Read the model definition and answer for the solid it produces. Units are mm, in the model's axes. Face numbers are marked on the shaded views. A direction names the side the tool comes from. Round coordinates to 2 decimals unless told otherwise and drop trailing zeros. Loops run counter-clockwise (first coordinate to the right, second up) from the corner with the lowest first, then second, coordinate; pieces in that order, holes last. Notation, with made-up numbers: M -9,74 L 6,74 A13 cw 6,94 Z; hole C -7.75,81 d5. An arc over 180 degrees is marked long. Answer as CSV lines item,"result".
Autodesk Inventor part; units mm, degrees
ref_plane "YZ Plane" through (0, 0, 0) normal (1, 0, 0) x (0, 1, 0)
ref_plane "XZ Plane" through (0, 0, 0) normal (0, 1, 0) x (-1, 0, 0)
ref_plane "XY Plane" through (0, 0, 0) normal (0, 0, 1) x (1, 0, 0)
sketch "Sketch1" plane through (0, 0, 0) normal (0, 0, 1) x (1, 0, 0)
  arc A0 (0.3627, 3.3303) -> (0.3911, -3.3271) centre (0, 0) ccw
  arc A1 (12.2334, -1.9351) -> (12.2164, 2.0395) centre (11.9999, 0.0513) ccw
  line L0 (0.3627, 3.3303) -> (12.2164, 2.0395)
  line L1 (12.2334, -1.9351) -> (0.3911, -3.3271)
  dimension "d0" = 6.7
  dimension "d2" = 4
  dimension "d3" = 12
extrude "Extrusion1" add sketch "Sketch1" against normal blind 1.3
sketch "Sketch2" plane through (0, 0, -1.3) normal (0, 0, -1) x (-1, 0, 0)
  arc A0 (-0.3911, -3.3271) -> (-0.3627, 3.3303) centre (0, 0) ccw
  circle A1 centre (0, 0) radius 3.35
  dimension "d6" = 6.7
extrude "Extrusion2" add sketch "Sketch2" along normal blind 3
sketch "Sketch3" plane through (0, 0, 0) normal (0, 0, 1) x (1, 0, 0)
  arc A0 (0.3627, 3.3303) -> (0.3911, -3.3271) centre (0, 0) ccw
hole "Hole1" at (0, 0, 0) direction (0, 0, -1) diameter 1.5 end through all counterbore diameter 3.8 counterbore depth 0.8
sketch "Sketch4" plane through (0, 0, -4.3) normal (0, 0, -1) x (-1, 0, 0)
  circle A0 centre (0, 0) radius 0.75
  circle A1 centre (0, 0) radius 3.35
  circle A2 centre (0, 0) radius 2
  dimension "d17" = 4
extrude "Extrusion3" cut sketch "Sketch4" against normal blind 3 contours A2
sketch "Sketch5" plane through (0, 0, 0) normal (0, 0, 1) x (1, 0, 0)
  arc A0 (12.2334, -1.9351) -> (12.2164, 2.0395) centre (11.9999, 0.0513) ccw
hole "Hole2" at (11.9999, 0.0513, 0) direction (0, 0, -1) diameter 2 end through all
properties part number "Servo Arm"
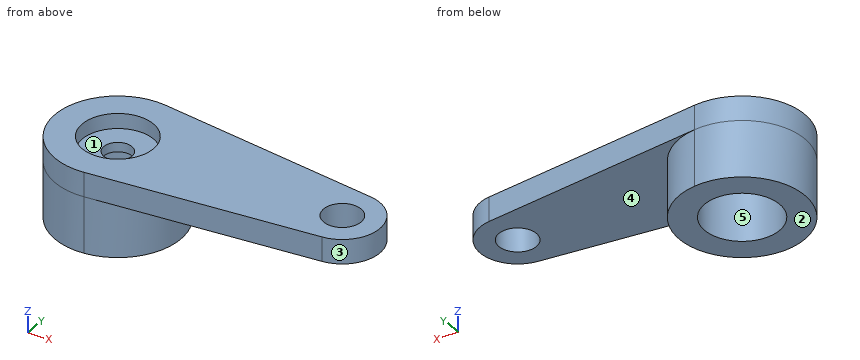
1) Find section B-B, the plane z = -2.6. Give the vertices of the cut face in (x, y), then the cut area to 3 significant figures.
Evaluation:
outline,"M 0.36,3.33 A3.35 ccw long 0.39,-3.33 A3.35 ccw Z; hole C 0,0 d4"
area,"22.7 mm^2"
2) Find section D-D, the plane y = -2.25. Give the vertices of the cut face in (x, z).
Evaluation:
outline,"M -2.48,-4.3 L 2.48,-4.3 L 2.48,-1.3 L 9.55,-1.3 L 9.55,0 L -2.48,0 Z"
3) Straight lines are drawn through the part: line 1 (X direction, y = 0, z = -1.05); line 2 (X direction, y = 0, z = -0.55); line 3 (Y direction, x = 0, z = -0.6). For each, find the intervals that lie inside material, in ascending order.
Evaluation:
line 1,"x = -3.35 to -0.75, 0.75 to 11, 13 to 14"
line 2,"x = -3.35 to -1.9, 1.9 to 11, 13 to 14"
line 3,"y = -3.35 to -1.9, 1.9 to 3.35"
4) Determine the mould class of the marked faces 3, 4 and 5 for opening direction X: released by +X, released by -X, zero draft, split by the parting line, or undercut.
Evaluation:
face 3,"released by +X"
face 4,"zero draft"
face 5,"undercut"
5) Find section C-C, the plane y = 0. Give the vertices of the cut face in (x, z), then the cut area to 3 significant figures.
Evaluation:
outline,"M -3.35,-4.3 L -2,-4.3 L -2,-1.3 L -0.75,-1.3 L -0.75,-0.8 L -1.9,-0.8 L -1.9,0 L -3.35,0 Z; M 0.75,-1.3 L 2,-1.3 L 2,-4.3 L 3.35,-4.3 L 3.35,-1.3 L 11,-1.3 L 11,0 L 1.9,0 L 1.9,-0.8 L 0.75,-0.8 Z; M 13,-1.3 L 14,-1.3 L 14,0 L 13,0 Z"
area,"24.3 mm^2"
6) A tool of negligible diameter and unlimited length cuts with its end or side. For the marked faces 1 and 2, from which of +Z, -Z, +X, -X, +Y, -Y can it reach the whole face along a straight path? Write none if from no direction.
Evaluation:
face 1,"+Z"
face 2,"-Z, +X, -X, +Y, -Y"
7) Each of these flat-tipped pins is pushed along its axis until it touches: P1, Ø1.5, axis at x = 9.5, y = -1, coming from the -Z side; P2, Ø1.7, axis at x = 0, y = 0, coming from the +Z side. Where does it stop, or does it pass through?
Evaluation:
P1,"stops at z = -1.3"
P2,"stops at z = -0.8"
8) Find section A-A, the plane x = 0. Give the vertices of the cut face in (y, z).
Evaluation:
outline,"M -3.35,-4.3 L -2,-4.3 L -2,-1.3 L -0.75,-1.3 L -0.75,-0.8 L -1.9,-0.8 L -1.9,0 L -3.35,0 Z; M 0.75,-1.3 L 2,-1.3 L 2,-4.3 L 3.35,-4.3 L 3.35,0 L 1.9,0 L 1.9,-0.8 L 0.75,-0.8 Z"
